For this review, take the finished solid that the model builds, in its own axes (mm). A direction names the side the tool comes from. Coordinates: 2 decimals unless noted, no trailing zeros. Loops run counter-clockwise (first coordinate to the right, second up) from the corner with the lowest first, then second, coordinate; pieces in that order, holes last. Notation, with made-up numbers: M 69.5,-23.75 L 96.5,-23.75 A22 cw 96.5,-5.75 Z; hole C 41,39.5 d8. An arc over 180 degrees is marked long. Write each question's results on one line, items separated by ' | '. Start each with the question number.
```python
from build123d import *

# Parameters (mm, degrees)
BOSS_EXTRUDE1_DEPTH = 3
SKETCH1_3_R         = 2.15
SKETCH1_3_R_2       = 1.6
SKETCH1_3_R_3       = 1.25
CUT_EXTRUDE1_DEPTH  = 71.818429805
BOSS_EXTRUDE2_START = 15
SKETCH1_4_R         = 1.25
BOSS_EXTRUDE2_DEPTH = 15
FILLET2_R           = 3
FILLET1_R           = 3


with BuildPart() as part:
    # Sketch1 → Boss-Extrude1 (new body)
    with BuildSketch(Plane(origin=(0, 0, 0), x_dir=(1, 0, 0), z_dir=(0, 1, 0))):
        with BuildLine():
            Line((-32.5, 60), (32.5, 60))
            ThreePointArc((32.5, 60), (36.035533906, 58.535533906), (37.5, 55))
            Line((37.5, 55), (37.5, -55))
            ThreePointArc((37.5, -55), (36.035533906, -58.535533906), (32.5, -60))
            Line((32.5, -60), (-32.5, -60))
            ThreePointArc((-32.5, -60), (-36.035533906, -58.535533906), (-37.5, -55))
            Line((-37.5, -55), (-37.5, 55))
            ThreePointArc((-37.5, 55), (-36.035533906, 58.535533906), (-32.5, 60))
        make_face()
    extrude(amount=-BOSS_EXTRUDE1_DEPTH)

    # Sketch1<3> → Cut-Extrude1 (cut, through all)
    with BuildSketch(Plane(origin=(0, 0, 0), x_dir=(1, 0, 0), z_dir=(0, 1, 0))):
        with Locations(Location((0, 51, 0), (0, 0, 270))):
            Circle(SKETCH1_3_R)
        with Locations(Location((0, -51, 0), (0, 0, 270))):
            Circle(SKETCH1_3_R)
        with Locations(Location((-29, -41, 0), (0, 0, 270))):
            Circle(SKETCH1_3_R_2)
        with Locations(Location((29, -41, 0), (0, 0, 270))):
            Circle(SKETCH1_3_R_2)
        with Locations(Location((29, 9, 0), (0, 0, 270))):
            Circle(SKETCH1_3_R_2)
        with Locations(Location((-29, 9, 0), (0, 0, 270))):
            Circle(SKETCH1_3_R_2)
        with Locations(Location((-19, 45, 0), (0, 0, 270))):
            Circle(SKETCH1_3_R_3)
        with Locations(Location((-19, 22, 0), (0, 0, 270))):
            Circle(SKETCH1_3_R_3)
        with Locations(Location((19, 22, 0), (0, 0, 90))):
            Circle(SKETCH1_3_R_3)
        with Locations(Location((19, 45, 0), (0, 0, 90))):
            Circle(SKETCH1_3_R_3)
    extrude(amount=-CUT_EXTRUDE1_DEPTH, mode=Mode.SUBTRACT)

    # Sketch1<4> → Boss-Extrude2 (add)
    # profile 1 of 4: a face of its own
    with BuildSketch(Plane(origin=(0, 0, 0), x_dir=(1, 0, 0), z_dir=(0, 1, 0)).offset(BOSS_EXTRUDE2_START)):
        with BuildLine():
            Line((-27, 42), (-19, 42))
            ThreePointArc((-19, 42), (-16, 45), (-19, 48))
            Line((-19, 48), (-27, 48))
            Line((-27, 48), (-27, 42))
        make_face()
        with Locations(Location((-19, 45, 0), (0, 0, 270))):
            Circle(SKETCH1_4_R, mode=Mode.SUBTRACT)
    # profile 2 of 4: a face of its own
    with BuildSketch(Plane(origin=(0, 0, 0), x_dir=(1, 0, 0), z_dir=(0, 1, 0)).offset(BOSS_EXTRUDE2_START)):
        with BuildLine():
            Line((-27, 19), (-19, 19))
            ThreePointArc((-19, 19), (-16, 22), (-19, 25))
            Line((-19, 25), (-27, 25))
            Line((-27, 25), (-27, 19))
        make_face()
        with Locations(Location((-19, 22, 0), (0, 0, 270))):
            Circle(SKETCH1_4_R, mode=Mode.SUBTRACT)
    # profile 3 of 4: a face of its own
    with BuildSketch(Plane(origin=(0, 0, 0), x_dir=(1, 0, 0), z_dir=(0, 1, 0)).offset(BOSS_EXTRUDE2_START)):
        with BuildLine():
            ThreePointArc((19, 19), (16, 22), (19, 25))
            Line((19, 25), (27, 25))
            Line((27, 25), (27, 19))
            Line((27, 19), (19, 19))
        make_face()
        with Locations(Location((19, 22, 0), (0, 0, 270))):
            Circle(SKETCH1_4_R, mode=Mode.SUBTRACT)
    # profile 4 of 4: a face of its own
    with BuildSketch(Plane(origin=(0, 0, 0), x_dir=(1, 0, 0), z_dir=(0, 1, 0)).offset(BOSS_EXTRUDE2_START)):
        with BuildLine():
            ThreePointArc((19, 42), (16, 45), (19, 48))
            Line((19, 48), (27, 48))
            Line((27, 48), (27, 42))
            Line((27, 42), (19, 42))
        make_face()
        with Locations(Location((19, 45, 0), (0, 0, 270))):
            Circle(SKETCH1_4_R, mode=Mode.SUBTRACT)
    extrude(amount=-BOSS_EXTRUDE2_DEPTH)

    # Fillet2
    fillet2_edges = [part.edges().sort_by_distance(p)[0] for p in [
        (-27, 7.5, -48),
        (-27, 7.5, -42),
        (-27, 7.5, -25),
        (-27, 7.5, -19),
        (27, 7.5, -19),
        (27, 7.5, -25),
        (27, 7.5, -48),
        (27, 7.5, -42),
    ]]
    fillet(fillet2_edges, radius=FILLET2_R - 0.0001)  # a hair under: the kernel refuses the full size

    # Fillet1
    fillet1_edges = [part.edges().sort_by_distance(p)[0] for p in [
        (16, 0, -22),
        (21.50005, 0, -25),
        (16, 0, -45),
        (21.50005, 0, -48),
        (-21.50005, 0, -42),
        (-21.50005, 0, -19),
        (21.50005, 0, -19),
        (21.50005, 0, -42),
        (-26.121349633, 0, -47.121349633),
        (-26.121349633, 0, -42.878650367),
        (-26.121349633, 0, -24.121349633),
        (-26.121349633, 0, -19.878650367),
        (26.121349633, 0, -19.878650367),
        (26.121349633, 0, -24.121349633),
        (26.121349633, 0, -47.121349633),
        (26.121349633, 0, -42.878650367),
        (-16, 0, -45),
        (-21.50005, 0, -48),
        (-16, 0, -22),
        (-21.50005, 0, -25),
    ]]
    fillet(fillet1_edges, radius=FILLET1_R)


solid = part.part
```
Q1. To check wall thickness, follow line 1 along X through (y, z) = (-1.55, -22); line 2 along Z through (x, y) = (19, -1.75); line 3 along X through (y, z) = (-2, -9). State the ranges of each line that lie inside material, in increasing order.
Q2. Insertion check: P1, Ø4, axis at x = 22, y = 9, coming from the -Z side; P2, Ø4, axis at x = -29, z = 41, coming from the +Y side; P3, Ø4, axis at x = -20.5, y = 10, coming from the +Z side. Each pin has a flat end and moves straight along its axis. Give the tip position at first contact, or say it passes through.
Q3. For faces 4 (the face through (-21.47, 0.9, -41.14)), 5 (the face through (0.65, -1.48, -48.95)), 6 (the face through (21, 9, -48)), 7 (the face through (-16, 9, -45)), list the 3-axis set-ups (+Z, -Z, +X, -X, +Y, -Y) from which the entire face can be reached by the end or side of a thin tool; tool diameter is ignored.
Q4. Take a section at B-B, the plane y = 5.5. Give the number of separate pieces and of enclosed holes in the cut face, then the cut area to 3 significant figures.
Q5. Take a section at A-A, the plane z = 41. Give the boundary of the cut face in (x, y).
Q6. Take a section at D-D, the plane x = 9. Give the boundary of the cut face in (y, z), then the cut area to 3 significant figures.
Q7. Take a section at C-C, the plane x = 0. Give the boundary of the cut face in (y, z).
Q8. The part is to be moulded in two halves that separate along Z. For faces 1 (the face through (26.14, 8.92, -47.1)), 2 (the face through (0.65, -1.48, 53.05)), 3 (the face through (-36, -1.48, 58.57)), say which applies: pulls with the +Z half, pulls with the -Z half, needs draft (parallel to the pull), parting line crosses it, or undercut.
Results:
1) line 1: -37.5 to -20.25, -17.75 to 17.75, 20.25 to 37.5 | line 2: -60 to -46.25, -43.75 to -23.25, -20.75 to 60 | line 3: -37.5 to -30.6, -27.4 to 27.4, 30.6 to 37.5
2) P1: z = -48 | P2: y = 0 | P3: z = -19
3) face 4: +X, -X, +Y | face 5: +Y, -Y | face 6: -Z, +X, -X, +Y | face 7: +Y
4) separate pieces: 4 | enclosed holes: 4 | area: 213 mm^2
5) outline: M -37.5,-3 L -30.6,-3 L -30.6,0 L -37.5,0 Z; M -27.4,-3 L 27.4,-3 L 27.4,0 L -27.4,0 Z; M 30.6,-3 L 37.5,-3 L 37.5,0 L 30.6,0 Z
6) outline: M -3,-60 L 0,-60 L 0,60 L -3,60 Z | area: 360 mm^2
7) outline: M -3,-60 L 0,-60 L 0,-53.15 L -3,-53.15 Z; M -3,-48.85 L 0,-48.85 L 0,48.85 L -3,48.85 Z; M -3,53.15 L 0,53.15 L 0,60 L -3,60 Z
8) face 1: pulls with the -Z half | face 2: undercut | face 3: pulls with the +Z half
